Job drawing, mm, ordinate dimensions from the low corner. One solid piece. A direction names the side the tool comes from. Give positions to 0.01 mm unless a question says otherwise; leave off trailing zeros. Write each loop counter-clockwise with the first axis right and the second up, starting at its lowest first coordinate (ties: lowest second). Pieces come first, ordered by that corner, then holes. Notation, with made-up numbers: (40.5, 89) - (92.5, 89) arc R30 ccw to (92.5, 116) - close; hole circle Ø4 at (58.5, 11). An arc over 180 degrees is marked (long way). Answer in a Markdown table with one row per item. Add a question column.
1. Band-saw the part on D-D on x = 10. Write the cut outline in (y, z), plus the area to 3 significant figures.
2. Probe line 1 along X through (y, z) = (31.15, 23); line 2 along X through (y, z) = (13.5, 5.5); line 3 along X through (y, z) = (19, 9.5). List the from-to ranges inside material, lowest first.
3. Band-saw the part on A-A on z = 16. Write the cut outline in (x, y).
4. Band-saw the part on C-C on y = 26. Write the cut outline in (x, z).
5. Which spindle directions (+Z, -Z, +X, -X, +Y, -Y) get a long thin tool onto all of the face, cutting with end or side? Do the marked faces 1, 2, 3, 4 and 5. Say none if no direction does.
6. Drop flat-ended pins along their axis: pin 1 Ø10 at (y, z) = (11, 7) entering from +X; pin 2 Ø6 at (x, z) = (8, 22.5) entering from -Y (1 decimal); pin 3 Ø2 at (y, z) = (11, 19) entering from -X; pin 4 Ø1.5 at (x, z) = (53, 12.5) entering from +Y (1 decimal). Give the stop position or say it passes through.
7. Band-saw the part on B-B on x = 28. Write the cut outline in (y, z), plus the area to 3 significant figures.
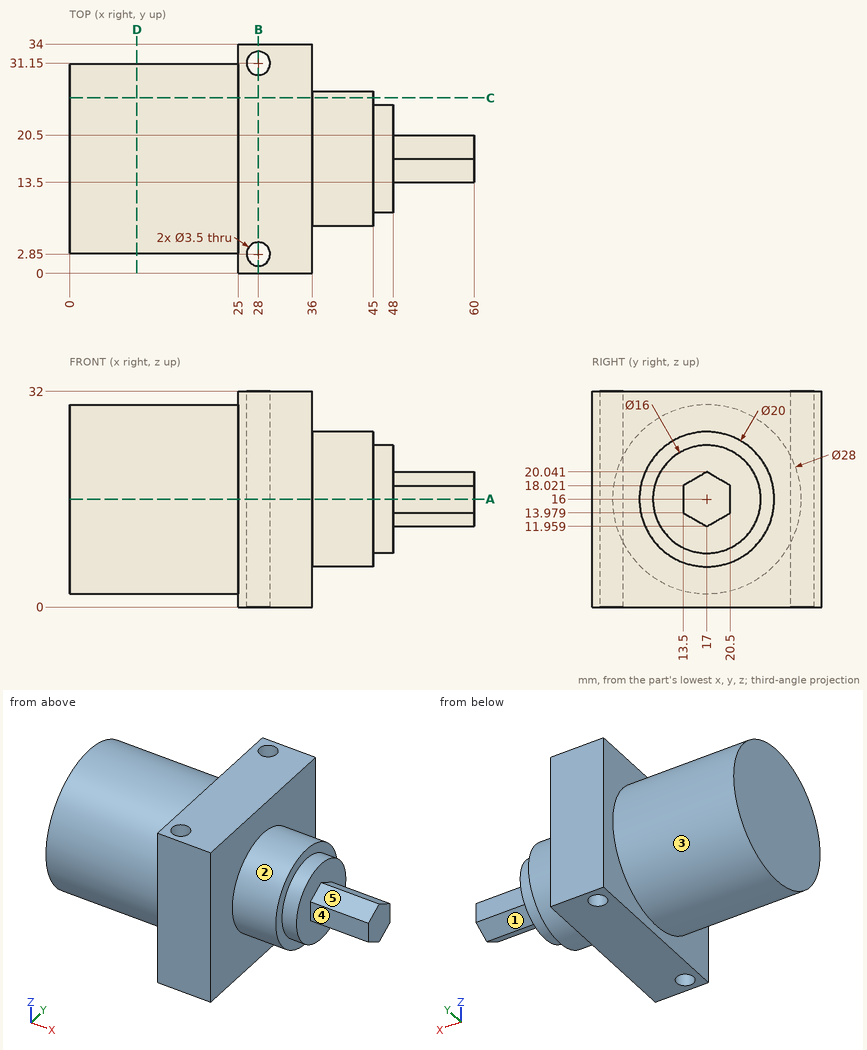
Values:
| question | item | result |
|---|---|---|
| 1 | outline | circle Ø28 at (17, 16) |
| 1 | area | 616 mm² |
| 2 | line 1 | x = 25 to 26.25, 29.75 to 36 |
| 2 | line 2 | x = 0 to 36 |
| 2 | line 3 | x = 0 to 48 |
| 3 | outline | (0, 3) - (25, 3) - (25, 0) - (36, 0) - (36, 7) - (45, 7) - (45, 9) - (48, 9) - (48, 13.5) - (60, 13.5) - (60, 20.5) - (48, 20.5) - (48, 25) - (45, 25) - (45, 27) - (36, 27) - (36, 34) - (25, 34) - (25, 31) - (0, 31) - close; hole circle Ø3.5 at (28, 2.85); hole circle Ø3.5 at (28, 31.15) |
| 4 | outline | (0, 5.28) - (25, 5.28) - (25, 0) - (36, 0) - (36, 11.64) - (45, 11.64) - (45, 20.36) - (36, 20.36) - (36, 32) - (25, 32) - (25, 26.72) - (0, 26.72) - close |
| 5 | face 1 | -Z, +X, +Y |
| 5 | face 2 | +X |
| 5 | face 3 | -X |
| 5 | face 4 | +Z, -Z, +X, -Y |
| 5 | face 5 | +Z, +X, -Y |
| 6 | pin 1 | stops at x = 48 |
| 6 | pin 2 | stops at y = 3.4 |
| 6 | pin 3 | stops at x = 0 |
| 6 | pin 4 | stops at y = 19.2 |
| 7 | outline | (0, 0) - (1.1, 0) - (1.1, 32) - (0, 32) - close; (4.6, 0) - (29.4, 0) - (29.4, 32) - (4.6, 32) - close; (32.9, 0) - (34, 0) - (34, 32) - (32.9, 32) - close |
| 7 | area | 864 mm² |
